Source: CAD feature listing. Evaluate the final solid. Frame: model axes, mm. A direction names the side the tool comes from. Give positions to 0.01 mm unless a question says otherwise; leave off trailing zeros. Write each loop counter-clockwise with the first axis right and the second up, starting at its lowest first coordinate (ties: lowest second). Pieces come first, ordered by that corner, then holes. Notation, with made-up numbers: M -16,-31.5 L 37,-31.5 A23 ccw 37,-3.5 Z; hole C 3.5,-2 d5. An arc over 180 degrees is marked long. Answer as a JSON object with one key per item and string values. Group by question number.
```python
from build123d import *

# Parameters (mm, degrees)
SKETCH_R           = 18
PAD_DEPTH          = 3
SKETCH001_R        = 15
PAD001_DEPTH       = 108
SKETCH002_R        = 9.5
PAD002_DEPTH       = 2.5
SKETCH003_R        = 13
PAD003_DEPTH       = 5.5
PAD004_DEPTH       = 1.5
POLARPATTERN_COUNT = 3
SKETCH009_W        = 8
SKETCH009_H        = 10
POCKET_DEPTH       = 118
SKETCH010_R        = 4.15
POCKET001_DEPTH    = 25
SKETCH011_R        = 4.3
POCKET002_DEPTH    = 25


with BuildPart() as part:
    # Sketch → Pad (new body)
    with BuildSketch(Plane.XY):
        Circle(SKETCH_R)
    extrude(amount=PAD_DEPTH)

    # Sketch001 (on Face3 of Pad) → Pad001 (join)
    with BuildSketch(Plane.XY.offset(3)):
        Circle(SKETCH001_R)
    extrude(amount=PAD001_DEPTH)

    # Sketch002 (on Face2 of Pad001) → Pad002 (join)
    with BuildSketch(Plane(origin=(0, 0, 0), x_dir=(1, 0, 0), z_dir=(0, 0, -1))):
        Circle(SKETCH002_R)
    extrude(amount=PAD002_DEPTH)

    # Sketch003 (on Face7 of Pad002) → Pad003 (join)
    with BuildSketch(Plane.XY.offset(111)):
        Circle(SKETCH003_R)
    extrude(amount=PAD003_DEPTH)

    # Sketch008 (on Face3 of Pad003) → Pad004 (join)
    with BuildSketch(Plane.XY.offset(3)):
        Polygon((-1.11579, 17.121659), (-0.012041, 17.758909), (1.091708, 17.121659), (1.091708, 15.84716), (-0.012041, 15.209911), (-1.11579, 15.84716), align=None)
    pad004 = extrude(amount=PAD004_DEPTH)

    # PolarPattern: Pad004 ×3 about axis
    polarpattern_axis = Axis((0, 0, 3), (0, 0, 1))
    for i in range(1, POLARPATTERN_COUNT):
        add(pad004.rotate(polarpattern_axis, i * 360 / POLARPATTERN_COUNT))

    # Sketch009 (on Face2 of PolarPattern) → Pocket (cut)
    with BuildSketch(Plane(origin=(0, 0, 0), x_dir=(1, 0, 0), z_dir=(0, 0, -1))):
        with Locations((-14, 0)):
            Rectangle(SKETCH009_W, SKETCH009_H)
    extrude(amount=-POCKET_DEPTH, mode=Mode.SUBTRACT)

    # Sketch010 (on Face7 of Pocket) → Pocket001 (cut)
    with BuildSketch(Plane(origin=(-10, 0, 0), x_dir=(0, -1, 0), z_dir=(-1, 0, 0))):
        with Locations((0, 36)):
            Circle(SKETCH010_R)
    extrude(amount=-POCKET001_DEPTH, mode=Mode.SUBTRACT)

    # Sketch011 → Pocket002 (cut)
    with BuildSketch(Plane(origin=(-10, 0, 0), x_dir=(0, -1, 0), z_dir=(-1, 0, 0))):
        with Locations((0, 60)):
            Circle(SKETCH011_R)
    extrude(amount=-POCKET002_DEPTH, mode=Mode.SUBTRACT)


solid = part.part
```
(1) Contact query for flat-ended pins moving along their axis: pin 1 Ø8 at (x, z) = (-13.5, 43) entering from +Y; pin 2 Ø0.7 at (x, y) = (-0.5, 16) entering from +Z; pin 3 Ø6 at (x, z) = (-13, 75) entering from +Y. Output: stop coordinate, or through.
(2) Ray query, L1, parallel to Z at x = 1, y = 0; L2, parallel to Z at x = 9.75, y = 0; L3, parallel to X at y = 0, z = 11.5. Return the intervals inside material, ascending. Write a range as [from, to].
(3) Section A-A, the plane y = 0. Return loops of the section in (x, z).
(4) Section D-D, the plane z = 16.5. Return loops of the section in (x, y), plus the area to 3 significant figures.
(5) Access query for faces 5 (the flat face through (12.04, -9.25, 3)), 6 (the flat face through (8, -8, 0)), 7 (the flat face through (-12, -5, 57)), 8 (the flat face through (14, -8, 4.5)). Directions: +Z, -Z, +X, -X, +Y, -Y. A direction counts if a zero-diameter tool reaches every point of the face in a straight line with its end or side. Return the directions, or none.
(6) Pull-direction query (Z, two-part tool) for faces 1 (the cylindrical face through (2.325, 0.56, 64.263)), 2 (the flat face through (0, 0, 116.5)), 3 (the cylindrical face through (2.33, -2.23, 39.5)), 4 (the flat face through (-10, -4, 57)); classes: pulls with the +Z half, pulls with the -Z half, needs draft (parallel to the pull), parting line crosses it, or undercut.
(7) Section B-B, the plane x = 8. Return loops of the section in (y, z), plus the area to 3 significant figures.
(8) Section C-C, the plane z = 60. Return loops of the section in (x, y), plus the area to 3 significant figures.
Reported:
{
 "1": {"pin 1": "stops at y = 11.61", "pin 2": "stops at z = 4.5", "pin 3": "stops at y = 11.18"},
 "2": {"L1": "z = [-2.5, 31.85], [40.15, 55.7], [64.3, 116.5]", "L2": "z = [0, 31.85], [40.15, 55.7], [64.3, 116.5]", "L3": "x = [-10, 15]"},
 "3": {"outline": "M -10,0 L -9.5,0 L -9.5,-2.5 L 9.5,-2.5 L 9.5,0 L 18,0 L 18,3 L 15,3 L 15,31.85 L -10,31.85 Z; M -10,40.15 L 15,40.15 L 15,55.7 L -10,55.7 Z; M -10,64.3 L 15,64.3 L 15,111 L 13,111 L 13,116.5 L -10,116.5 Z"},
 "4": {"outline": "M -14.14,-5 A15 ccw long -14.14,5 L -10,5 L -10,-5 Z", "area": "660 mm2"},
 "5": {"face 5": "+Z", "face 6": "-Z", "face 7": "+Z, -Z, -X", "face 8": "+Z, +X, -Y"},
 "6": {"face 1": "undercut", "face 2": "pulls with the +Z half", "face 3": "undercut", "face 4": "needs draft"},
 "7": {"outline": "M -16.12,0 L -5.12,0 L -5.12,-2.5 L 5.12,-2.5 L 5.12,0 L 16.12,0 L 16.12,3 L 12.69,3 L 12.69,111 L 10.25,111 L 10.25,116.5 L -10.25,116.5 L -10.25,111 L -12.69,111 L -12.69,3 L -16.12,3 Z; hole C 0,60 d8.6; hole C 0,36 d8.3", "area": "2,860 mm2"},
 "8": {"outline": "M -14.14,-5 A15 ccw 14.37,-4.3 L -10,-4.3 L -10,-5 Z; M -14.14,5 L -10,5 L -10,4.3 L 14.37,4.3 A15 ccw Z", "area": "446 mm2"}
}
